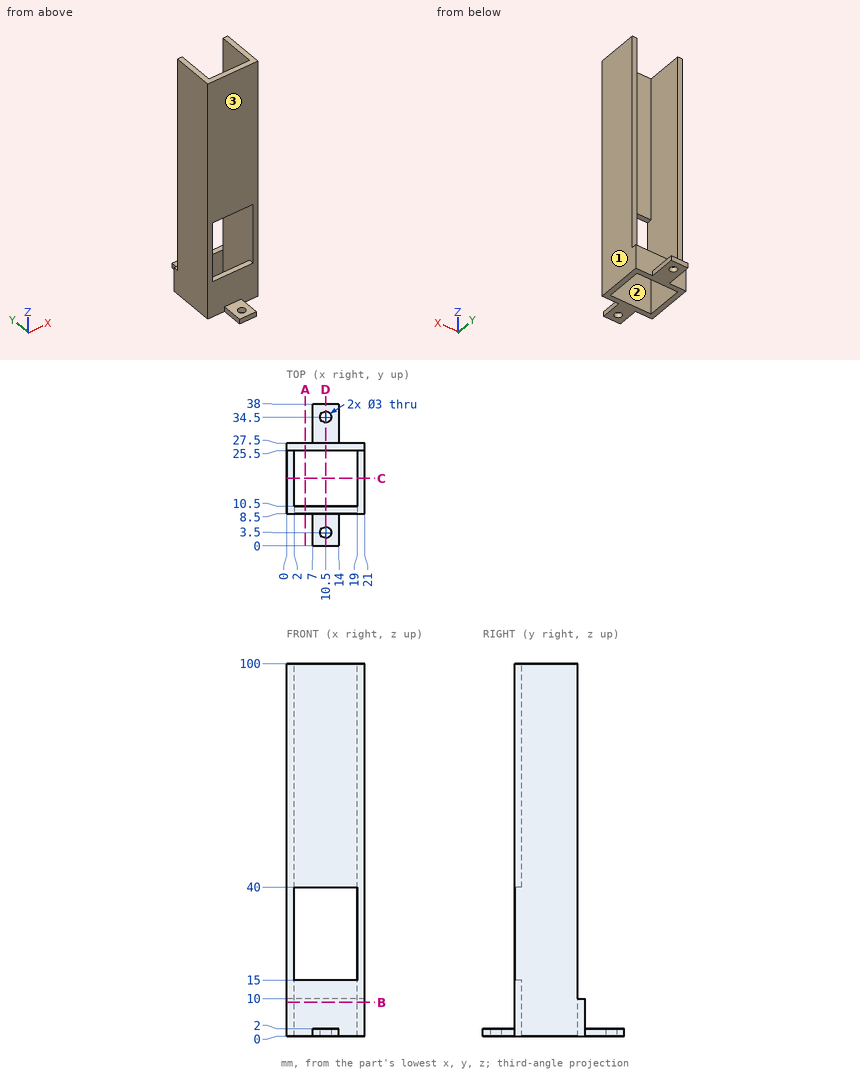
Answer from the drawing. Dimensions are ordinates in mm from the lowest x, y and z of the part. Coordinates: 2 decimals unless noted, no trailing zeros. Write each loop counter-clockwise with the first axis right and the second up, starting at its lowest first coordinate (ties: lowest second). Pieces come first, ordered by that corner, then holes. Notation, with made-up numbers: M 25.25,19 L 83.25,19 A32 ccw 83.25,47 Z; hole C -20,-23 d9. An arc over 180 degrees is marked long. Put each result on its own line as item: value. Start each with the question number.
1. A cutting plane is placed at B-B on z = 9. Write down the section's boundary in (x, y).
2. Flat-ended cylindrical pins translate along their axes: P1, Ø6, axis at x = 6, z = 71, coming from the +Y side; P2, Ø2, axis at x = 10, y = 32, coming from the +Z side; P3, Ø4, axis at x = 12, z = 87, coming from the -Y side; P4, Ø1, axis at x = 8, y = 9, coming from the -Z side. Find the tip coordinate at first contact, or state that the pin passes through.
3. A cutting plane is placed at A-A on x = 5. Write down the section's boundary in (y, z).
4. A cutting plane is placed at D-D on x = 10.5. Write down the section's boundary in (y, z).
5. Consider line 1 (Y direction, x = 10.5, z = 0.8); line 2 (Y direction, x = 2.5, z = 6.5); line 3 (X direction, y = 34, z = 1). Determine where each line is inside the solid, lowest interval first. Write a range as from..to.
6. For a pull along X with two mould halves and no side action, classify the marked faces 1, 2 and 3 as pulls with the +X half, pulls with the -X half, needs draft (parallel to the pull), parting line crosses it, or undercut.
7. A cutting plane is placed at C-C on y = 18. Write down the section's boundary in (x, z), then the cut area to 3 significant figures.
Resolved:
1. outline: M 0,8.5 L 21,8.5 L 21,27.5 L 0,27.5 Z; hole M 2,10.5 L 19,10.5 L 19,25.5 L 2,25.5 Z
2. P1: stops at y = 10.5
2. P2: stops at z = 2
2. P3: stops at y = 8.5
2. P4: stops at z = 0
3. outline: M 8.5,0 L 10.5,0 L 10.5,15 L 8.5,15 Z; M 8.5,40 L 10.5,40 L 10.5,100 L 8.5,100 Z; M 25.5,0 L 27.5,0 L 27.5,10 L 25.5,10 Z
4. outline: M 0,0 L 2,0 L 2,2 L 0,2 Z; M 5,0 L 10.5,0 L 10.5,15 L 8.5,15 L 8.5,2 L 5,2 Z; M 8.5,40 L 10.5,40 L 10.5,100 L 8.5,100 Z; M 25.5,0 L 33,0 L 33,2 L 27.5,2 L 27.5,10 L 25.5,10 Z; M 36,0 L 38,0 L 38,2 L 36,2 Z
5. line 1: y = 0..2, 5..10.5, 25.5..33, 36..38
5. line 2: y = 8.5..10.5, 25.5..27.5
5. line 3: x = 7..9.09, 11.91..14
6. face 1: pulls with the +X half
6. face 2: undercut
6. face 3: needs draft
7. outline: M 0,0 L 2,0 L 2,100 L 0,100 Z; M 19,0 L 21,0 L 21,100 L 19,100 Z
7. area: 400 mm2
